Source: CAD feature listing. Evaluate the final solid. Frame: model axes, mm. Face numbers are marked on the shaded views. Give positions to 0.01 mm unless a question says otherwise; leave off trailing zeros. Order: outer loops, then holes, each group sorted by start corner. A loop starts at its lowest first (then second) coordinate and runs counter-clockwise, first axis right, second up. Notation, with made-up numbers: (66, 77) -> (86, 77) arc R26 cw to (86, 103) -> close; hole circle Ø2 at (4.25, 71.25). An arc over 180 degrees is marked (long way). Use one line per item in the form item = value. Start each with the question number.
from build123d import *

# Parameters (mm, degrees)
F1_DEPTH      = 711.2
F3_DEPTH      = 50.801
F3_DEPTH_BACK = 50.801
F5_DEPTH      = 50.801
F5_DEPTH_BACK = 50.801


with BuildPart() as f1:
    # F0 (on Top) → F1 (new body)
    with BuildSketch(Plane.XY):
        with BuildLine():
            Line((-22.225, -50.8), (22.225, -50.8))
            ThreePointArc((22.225, -50.8), (24.4700640303, -49.8700640303), (25.4, -47.625))
            Line((25.4, -47.625), (25.4, 47.625))
            ThreePointArc((25.4, 47.625), (24.4700640303, 49.8700640303), (22.225, 50.8))
            Line((22.225, 50.8), (-22.225, 50.8))
            ThreePointArc((-22.225, 50.8), (-24.4700640303, 49.8700640303), (-25.4, 47.625))
            Line((-25.4, 47.625), (-25.4, -47.625))
            ThreePointArc((-25.4, -47.625), (-24.4700640303, -49.8700640303), (-22.225, -50.8))
        make_face()
        with BuildLine():
            ThreePointArc((22.225, -44.45), (21.2950640303, -46.6950640303), (19.05, -47.625))
            Line((19.05, -47.625), (-19.05, -47.625))
            ThreePointArc((-19.05, -47.625), (-21.2950640303, -46.6950640303), (-22.225, -44.45))
            Line((-22.225, -44.45), (-22.225, 44.45))
            ThreePointArc((-22.225, 44.45), (-21.2950640303, 46.6950640303), (-19.05, 47.625))
            Line((-19.05, 47.625), (19.05, 47.625))
            ThreePointArc((19.05, 47.625), (21.2950640303, 46.6950640303), (22.225, 44.45))
            Line((22.225, 44.45), (22.225, -44.45))
        make_face(mode=Mode.SUBTRACT)
    extrude(amount=F1_DEPTH)

    # F2 (on Front) → F3 (cut, two sides)
    with BuildSketch(Plane.XZ) as f3_sk:
        Polygon((25.4, 18.4896879007), (-25.4, 0), (25.4, 0), align=None)
    extrude(amount=-F3_DEPTH, mode=Mode.SUBTRACT)
    extrude(f3_sk.sketch, amount=F3_DEPTH_BACK, mode=Mode.SUBTRACT)

    # F4 (on Front) → F5 (cut, two sides)
    with BuildSketch(Plane.XZ) as f5_sk:
        Polygon((25.4, 711.2), (-25.4, 711.2), (25.4, 675.6294570589), align=None)
    extrude(amount=-F5_DEPTH, mode=Mode.SUBTRACT)
    extrude(f5_sk.sketch, amount=F5_DEPTH_BACK, mode=Mode.SUBTRACT)


solid = f1.part
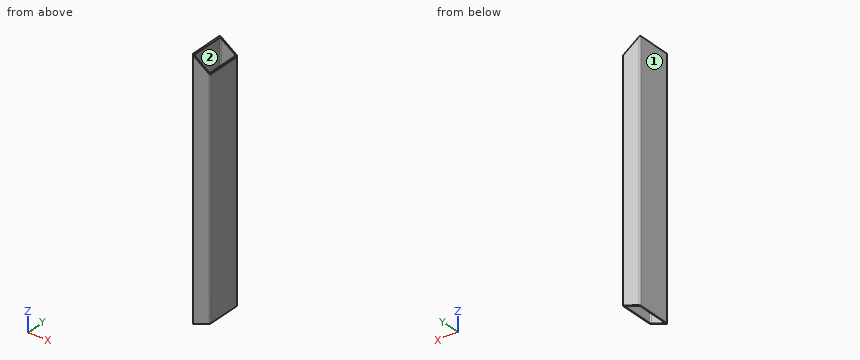
1) Cut plane B-B, the plane x = -8. Return the cut outline in (y, z) (3 decimals).
2) Material intervals for probe 1 along X at (y, z) = (29.5, 656) (3 decimals); probe 2 along Y at (x, z) = (-16, 131.5) (3 decimals); probe 3 along Y at (x, z) = (-20.5, 512), sorted ascending.
3) Cut plane C-C, the plane z = 430. Return the cut outline in (x, y) (3 decimals).
4) Draft query along Y for the marked faces 1 and 2. Return one class per face: +Y half, -Y half, draft (parallel to the pull), parting line (faces both ways), or undercut.
5) Cut plane A-A, the plane y = 25. Return the cut outline in (x, z) (3 decimals).
Output values:
q1.outline = (-50.8, 6.333) -> (-47.625, 6.333) -> (-47.625, 699.016) -> (-50.8, 699.016) -> close; (47.625, 6.333) -> (50.8, 6.333) -> (50.8, 699.016) -> (47.625, 699.016) -> close
q2.probe_1 = -25.4 to -22.225, 22.225 to 25.4
q2.probe_2 = -50.8 to -47.625, 47.625 to 50.8
q2.probe_3 = -50.8 to -47.27, 47.27 to 50.8
q3.outline = (-25.4, -47.625) arc R3.175 ccw to (-22.225, -50.8) -> (22.225, -50.8) arc R3.175 ccw to (25.4, -47.625) -> (25.4, 47.625) arc R3.175 ccw to (22.225, 50.8) -> (-22.225, 50.8) arc R3.175 ccw to (-25.4, 47.625) -> close; hole (-22.225, -44.45) arc R3.175 ccw to (-19.05, -47.625) -> (19.05, -47.625) arc R3.175 ccw to (22.225, -44.45) -> (22.225, 44.45) arc R3.175 ccw to (19.05, 47.625) -> (-19.05, 47.625) arc R3.175 ccw to (-22.225, 44.45) -> close
q4.face_1 = draft
q4.face_2 = undercut
q5.outline = (-25.4, 0) -> (-22.225, 1.156) -> (-22.225, 708.977) -> (-25.4, 711.2) -> close; (22.225, 17.334) -> (25.4, 18.49) -> (25.4, 675.629) -> (22.225, 677.853) -> close
